from build123d import *

# Parameters (mm, degrees)
F0_R     = 4.5
F1_DEPTH = 10
F2_W     = 5
F2_H     = 5
F3_DEPTH = 10
F4_SIZE  = 4.99999
F5_DEPTH = 10
F7_D     = 2
F7_DEPTH = 9
F7_TIP   = 0.600860619


# Not quite as in the source:
# - a fillet or chamfer is up to 0.001 mm smaller than in the source, because OpenCascade refuses the exact size


with BuildPart() as f1:
    # F0 (on Top) → F1 (new body)
    with BuildSketch(Plane.XY):
        Circle(F0_R)
    extrude(amount=F1_DEPTH)

    # F2 (on face) → F3 (join)
    with BuildSketch(Plane.XY.offset(10)):
        with BuildLine():
            ThreePointArc((2.5, -3.7416573868), (0, -4.5), (-2.5, -3.7416573868))
            Line((-2.5, -3.7416573868), (-2.5, -20))
            Line((-2.5, -20), (2.5, -20))
            Line((2.5, -20), (2.5, -3.7416573868))
        make_face()
        with BuildLine():
            Line((-3.7416573868, 2.5), (-20, 2.5))
            Line((-20, 2.5), (-20, -2.5))
            Line((-20, -2.5), (-3.7416573868, -2.5))
            ThreePointArc((-3.7416573868, -2.5), (-4.5, 0), (-3.7416573868, 2.5))
        make_face()
        with BuildLine():
            Line((-2.5, 20), (-2.5, 3.7416573868))
            ThreePointArc((-2.5, 3.7416573868), (0, 4.5), (2.5, 3.7416573868))
            Line((2.5, 3.7416573868), (2.5, 20))
            Line((2.5, 20), (-2.5, 20))
        make_face()
        with BuildLine():
            Line((20, 2.5), (3.7416573868, 2.5))
            ThreePointArc((3.7416573868, 2.5), (4.3062430401, 1.3062430401), (4.5, 0))
            ThreePointArc((4.5, 0), (4.3062430401, -1.3062430401), (3.7416573868, -2.5))
            Line((3.7416573868, -2.5), (20, -2.5))
            Line((20, -2.5), (20, 2.5))
        make_face()
        with BuildLine():
            Line((3.7416573868, 2.5), (2.5, 2.5))
            Line((2.5, 2.5), (2.5, -2.5))
            Line((2.5, -2.5), (3.7416573868, -2.5))
            ThreePointArc((3.7416573868, -2.5), (4.3062430401, -1.3062430401), (4.5, 0))
            ThreePointArc((4.5, 0), (4.3062430401, 1.3062430401), (3.7416573868, 2.5))
        make_face()
        Rectangle(F2_W, F2_H)
        with BuildLine():
            Line((2.5, -2.5), (-2.5, -2.5))
            Line((-2.5, -2.5), (-2.5, -3.7416573868))
            ThreePointArc((-2.5, -3.7416573868), (0, -4.5), (2.5, -3.7416573868))
            Line((2.5, -3.7416573868), (2.5, -2.5))
        make_face()
        with BuildLine():
            Line((-2.5, 2.5), (-3.7416573868, 2.5))
            ThreePointArc((-3.7416573868, 2.5), (-4.5, 0), (-3.7416573868, -2.5))
            Line((-3.7416573868, -2.5), (-2.5, -2.5))
            Line((-2.5, -2.5), (-2.5, 2.5))
        make_face()
        with BuildLine():
            Line((-2.5, 3.7416573868), (-2.5, 2.5))
            Line((-2.5, 2.5), (2.5, 2.5))
            Line((2.5, 2.5), (2.5, 3.7416573868))
            ThreePointArc((2.5, 3.7416573868), (0, 4.5), (-2.5, 3.7416573868))
        make_face()
    extrude(amount=F3_DEPTH)

    # F4 (size 5 in the source; OpenCascade refuses exactly that, so slightly less here)
    f4_edges = [f1.edges().sort_by_distance(p)[0] for p in [
        (-2.5, -11.25, 20),
        (-11.25, 2.5, 20),
        (2.5, 11.25, 20),
        (11.25, -2.5, 20),
    ]]
    chamfer(f4_edges, length=F4_SIZE)

    # F5 (add): faces of the model
    f5_faces = [f1.faces().sort_by_distance(p)[0] for p in [
        (-2.940797231, 2.940797231, 10),
        (2.940797231, 2.940797231, 10),
        (2.940797231, -2.940797231, 10),
        (-2.940797231, -2.940797231, 10),
    ]]
    extrude(f5_faces, amount=F5_DEPTH)

    # F7
    with Locations(Plane(origin=(0, 0, 0), x_dir=(1, 0, 0), z_dir=(0, 0, -1))):
        with Locations((0, 0)):
            Hole(F7_D / 2, depth=F7_DEPTH)
            with Locations((0, 0, -(F7_DEPTH + F7_TIP / 2))):  # 118° drill point
                Cone(0, F7_D / 2, F7_TIP, mode=Mode.SUBTRACT)


solid = f1.part
Here's how the part is built. I have some questions about the finished solid (model axes, mm). A direction names the side the tool comes from. Round coordinates to 2 decimals unless told otherwise and drop trailing zeros. Order: outer loops, then holes, each group sorted by start corner. A loop starts at its lowest first (then second) coordinate and runs counter-clockwise, first axis right, second up. Notation, with made-up numbers: M -14.75,23.5 L 13.25,23.5 A21 ccw 13.25,36.5 Z; hole C -28,-10 d2. An arc over 180 degrees is marked long. Return JSON: item names as keys, results as strings. Group by question number.
1. If we section it at B-B on z = 13: List the corners of the cut face in (x, y) for me, then the cut area to 3 significant figures.
2. Please list where these lines run through material, in increasing order: probe 1 along Y at (x, z) = (0, 4.75); probe 2 along Y at (x, z) = (12, 16.5); probe 3 along Y at (x, z) = (-11.5, 11.5).
3. If we mould it in two halves opening along Y, with no side actions, what happens to faces 6 (the face through (2.5, 12, 12)), 7 (the face through (3, -2.5, 17)), 8 (the face through (12, 2.5, 15))? For each: pulls with the +Y half, pulls with the -Y half, needs draft (parallel to the pull), parting line crosses it, or undercut.
4. I'm going to push flat-ended pins straight in: pin 1 Ø12 at (y, z) = (5, 2.5) entering from +X; pin 2 Ø5.5 at (y, z) = (0.5, 18.5) entering from -X; pin 3 Ø4 at (x, y) = (11.5, -1) entering from -Z; pin 4 Ø4 at (x, z) = (-8.5, 12) entering from +Y. Where does each tip first touch, or does it pass through?
5. On a 3-axis mill with a long thin cutter (end or side, diameter ignored), from which of +Z, -Z, +X, -X, +Y, -Y can I reach the whole of each face in a straight line? I mean faces 1 (the face through (12, -2.5, 12)), 2 (the face through (-12, -2.5, 15)), 3 (the face through (-2.5, -3, 17)), 4 (the face through (2.5, -1, 19)), 5 (the face through (-3, 2.5, 17)). Say none if no direction works.
Reply:
{
 "1": {"outline": "M -20,-2.5 L -3.74,-2.5 A4.5 ccw -2.5,-3.74 L -2.5,-20 L 2.5,-20 L 2.5,-3.74 A4.5 ccw 3.74,-2.5 L 20,-2.5 L 20,2.5 L 3.74,2.5 A4.5 ccw 2.5,3.74 L 2.5,20 L -2.5,20 L -2.5,3.74 A4.5 ccw -3.74,2.5 L -20,2.5 Z", "area": "378 mm^2"},
 "2": {"probe 1": "-4.5 to -1, 1 to 4.5", "probe 2": "-1 to 2.5", "probe 3": "-2.5 to 2.5"},
 "3": {"face 6": "needs draft", "face 7": "undercut", "face 8": "pulls with the +Y half"},
 "4": {"pin 1": "x = 4.5", "pin 2": "x = -20", "pin 3": "z = 10", "pin 4": "y = 2.5"},
 "5": {"face 1": "+Z, -Z, +X, -Y", "face 2": "+Z, -Z, -X, -Y", "face 3": "+Z, -Y", "face 4": "+Z, +X", "face 5": "+Z, -X"}
}
